Autodesk Inventor part; units mm, degrees
ref_plane "Plano de trabalho4" through (29, 0, 0) normal (1, 0, 0) x (0, 1, 0)
ref_plane "XZ Plane" through (0, 0, 0) normal (0, 1, 0) x (-1, 0, 0)
ref_plane "XY Plane" through (0, 0, 0) normal (0, 0, 1) x (1, 0, 0)
sketch "Esboço1" plane through (0, 0, 0) normal (0, 0, 1) x (1, 0, 0)
  circle A0 centre (0, 0) radius 14.5
  dimension "d0" = 29
extrude "Extrusão1" add sketch "Esboço1" along normal blind 2
sketch "Esboço2" plane through (0, 0, 2) normal (0, 0, 1) x (1, 0, 0)
  circle A0 centre (0, 0) radius 14.5
  circle A1 centre (0, 0) radius 12.5
  dimension "d3" = 2
extrude "Extrusão2" add sketch "Esboço2" along normal blind 58
ref_plane "Plano de trabalho4" through (29, 0, 0) normal (1, 0, 0) x (0, 1, 0)
sketch "Esboço5" plane through (29, 0, 0) normal (1, 0, 0) x (0, 1, 0)
  line L0 (-7.75, 27) -> (7.75, 27)
  line L1 (7.75, 27) -> (7.75, 6.5)
  line L2 (7.75, 6.5) -> (-7.75, 6.5)
  line L3 (-7.75, 6.5) -> (-7.75, 27)
  line L4 (-7.75, 27) -> (7.75, 6.5) construction
  line L5 (7.75, 27) -> (-7.75, 6.5) construction
  line L6 (14.5, 0) -> (-14.5, 0)
  point P0 (0, 0)
  point P1 (0, 16.75)
  dimension "d15" = 20.5
  dimension "d16" = 15.5
  dimension "d17" = 0
  dimension "d18" = 6.5
extrude "Extrusão4" cut sketch "Esboço5" against normal through all
sketch "Esboço7" plane through (0, 0, 60) normal (0, 0, 1) x (1, 0, 0)
  circle A0 centre (0, 0) radius 16.5
  circle A1 centre (0, 0) radius 12.5
  dimension "d28" = 33
extrude "Extrusão6" add sketch "Esboço7" along normal blind 2
fillet "Arredondamento2" radius 2 1 edges at (-12.5, 0, 62)
fillet "Arredondamento3" radius 2 1 edges at (-14.5, 0, 60)
sketch "Sketch8" plane through (0, 0, 0) normal (1, 0, 0) x (0, 1, 0)
  line L0 (-9.75, 23.25) -> (9.75, 23.25)
  line L1 (9.75, 23.25) -> (9.75, 25)
  line L2 (9.75, 25) -> (-9.75, 25)
  line L3 (-9.75, 25) -> (-9.75, 23.25)
  line L4 (-7.75, 27) -> (7.75, 27)
  line L5 (7.75, 27) -> (7.75, 6.5)
  line L6 (-7.75, 6.5) -> (-7.75, 27)
  point P0 (0, 0)
  dimension "d37" = 2
  dimension "d38" = 1.75
  dimension "d39" = 2
  dimension "d40" = 2
extrude "Extrusion7" cut sketch "Sketch8" along normal mid plane 50 contours L3 L2 L6 L0 | L6 L2 L5 L0 | L5 L2 L1 L0
Work out the finished part from the listing and answer in its coordinate system (mm). A direction names the side the tool comes from. Coordinates: 2 decimals unless noted, no trailing zeros. Write each loop counter-clockwise with the first axis right and the second up, starting at its lowest first coordinate (ties: lowest second). Pieces come first, ordered by that corner, then holes. Notation, with made-up numbers: M 70,17.5 L 89,17.5 A34 ccw 89,47.5 Z; hole C -16.5,62.5 d5. An arc over 180 degrees is marked long. Use one line per item in the form item = value. Start each with the question number.
1. The mould has two halves that part along Y. Classify faces 1 (the face through (6.72, -10.54, 30.59)), 2 (the face through (0, -15, 62)), 3 (the face through (15.24, 6.32, 60.99)): released by +Y, released by -Y, zero draft, split by the parting line, or undercut.
2. Straight lines are drawn through the part: probe 1 along Y at (x, z) = (0, 47); probe 2 along Z at (x, y) = (9, 8.5); probe 3 along Y at (x, z) = (-10.5, 12). For each, find the intervals that lie inside material, in ascending order. Write a range as from..to.
3. The part is cut by section A-A (y = 0). Give the number of separate pieces and of enclosed holes in the cut face, plus the area to 3 significant figures.
4. Each of these flat-tipped pins is pushed along its axis until it touches: P1, Ø1.6, axis at x = -11.5, z = 26.5, coming from the -Y side; P2, Ø2, axis at x = -9.5, y = -8.5, coming from the +Z side; P3, Ø10, axis at x = 11.5, y = -8.5, coming from the +Z side; P4, Ø3, axis at x = 3, z = 39.5, coming from the +Y side. Where does it stop, or does it pass through?
5. The part is cut by section D-D (z = 28). Give the vertices of the cut face in (x, y).
6. The part is cut by section B-B (z = 10). Give the vertices of the cut face in (x, y).
7. A tool of negligible diameter and unlimited length cuts with its end or side. For faces 4 (the face through (11, 7.75, 15)), 5 (the face through (-14.486, -0.638, 28.594)), from which of +Z, -Z, +X, -X, +Y, -Y can it reach the whole face along a straight path? Write none if from no direction.
Evaluation:
q1.face_1 = undercut
q1.face_2 = zero draft
q1.face_3 = split by the parting line
q2.probe_1 = -14.5..-12.5, 12.5..14.5
q2.probe_2 = 0..2
q2.probe_3 = -10..-7.75, 7.75..10
q3.separate_pieces = 3
q3.enclosed_holes = 0
q3.area = 224 mm^2
q4.P1 = -9.79
q4.P2 = 61.85
q4.P3 = 62
q4.P4 = 14.42
q5.outline = C 0,0 d29; hole C 0,0 d25
q6.outline = M -12.26,-7.75 A14.5 ccw 12.26,-7.75 L 9.81,-7.75 A12.5 cw -9.81,-7.75 Z; M -12.26,7.75 L -9.81,7.75 A12.5 cw 9.81,7.75 L 12.26,7.75 A14.5 ccw Z
q7.face_4 = +X, -X
q7.face_5 = -Z
